Geometry check sheet. Reference: the model listing, model coordinates, mm. Face numbers are marked on the shaded views. A direction names the side the tool comes from. Round coordinates to 2 decimals unless told otherwise and drop trailing zeros. Order: outer loops, then holes, each group sorted by start corner. A loop starts at its lowest first (then second) coordinate and runs counter-clockwise, first axis right, second up.
(1) Set-up check for the marked faces 1, 2 and 3: record each of +Z, -Z, +X, -X, +Y, -Y from which the full face is reachable in a straight line by a thin tool's end or side.
(2) Sectioned sample at A-A (z = 0). Record the boundary of the cut face in (x, y).
(3) Material ranges on line 1 along X through (y, z) = (-10.5, 0); line 2 along X through (y, z) = (5, -4.5); line 3 along Z through (x, y) = (-216, 10), recorded low to high.
(4) Sectioned sample at B-B (y = 0). Record the boundary of the cut face in (x, z).
(5) Go/stop test with flat-tipped pins: pin 1 (6 mm diameter, centred on x = 0.5, y = -14, fed in from +Z); pin 2 (3 mm diameter, centred on x = 128.5, y = -12, fed in from +Z); pin 3 (8 mm diameter, centred on x = -22, y = 7, fed in from +Z). Record where each tip stops, or that it passes through.
(6) Sectioned sample at C-C (x = -216). Record the boundary of the cut face in (y, z).
(7) Sectioned sample at D-D (x = 181.5). Record the boundary of the cut face in (y, z), plus the area to 3 significant figures.
from build123d import *

# Parameters (mm, degrees)
F0_R     = 18.5
F1_DEPTH = 268.5
F2_R     = 5
F3_DEPTH = 25
F4_SIZE  = 2
F5_R     = 21
F6_DEPTH = 173


with BuildPart() as f1:
    # F0 (on Right) → F1 (new body, symmetric)
    with BuildSketch(Plane.YZ):
        Circle(F0_R)
    extrude(amount=F1_DEPTH, both=True)

    # F2 (on Front) → F3 (cut, symmetric)
    with BuildSketch(Plane.XZ):
        with Locations((-216, 0)):
            Circle(F2_R)
        with Locations((216, 0)):
            Circle(F2_R)
    extrude(amount=F3_DEPTH, both=True, mode=Mode.SUBTRACT)

    # F4
    f4_edges = [f1.edges().sort_by_distance(p)[0] for p in [
        (-268.5, -18.5, 0),
        (268.5, -18.5, 0),
    ]]
    chamfer(f4_edges, length=F4_SIZE)

    # F5 (on Right) → F6 (join, symmetric)
    with BuildSketch(Plane.YZ):
        Circle(F5_R)
    extrude(amount=F6_DEPTH, both=True)


solid = f1.part
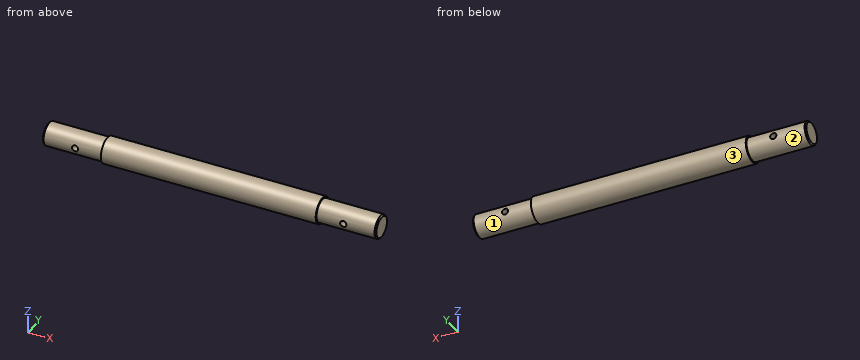
Answer below:
1. face 1: +X
1. face 2: -X
1. face 3: +X, -X
2. outline: (-268.5, -16.5) - (-266.5, -18.5) - (-221, -18.5) - (-221, 18.5) - (-266.5, 18.5) - (-268.5, 16.5) - close; (-211, -18.5) - (-173, -18.5) - (-173, -21) - (173, -21) - (173, -18.5) - (211, -18.5) - (211, 18.5) - (173, 18.5) - (173, 21) - (-173, 21) - (-173, 18.5) - (-211, 18.5) - close; (221, -18.5) - (266.5, -18.5) - (268.5, -16.5) - (268.5, 16.5) - (266.5, 18.5) - (221, 18.5) - close
3. line 1: x = -268.5 to -221, -211 to 211, 221 to 268.5
3. line 2: x = -268.5 to -218.18, -213.82 to 213.82, 218.18 to 268.5
3. line 3: z = -15.56 to -5, 5 to 15.56
4. outline: (-268.5, -16.5) - (-266.5, -18.5) - (-173, -18.5) - (-173, -21) - (173, -21) - (173, -18.5) - (266.5, -18.5) - (268.5, -16.5) - (268.5, 16.5) - (266.5, 18.5) - (173, 18.5) - (173, 21) - (-173, 21) - (-173, 18.5) - (-266.5, 18.5) - (-268.5, 16.5) - close; hole circle Ø10 at (-216, 0); hole circle Ø10 at (216, 0)
5. pin 1: stops at z = 17.89
5. pin 2: stops at z = 18.19
5. pin 3: stops at z = 20.78
6. outline: (-17.81, -5) arc R18.5 ccw to (17.81, -5) - close; (-17.81, 5) - (17.81, 5) arc R18.5 ccw to start
7. outline: circle Ø37 at (0, 0)
7. area: 1,080 mm2
